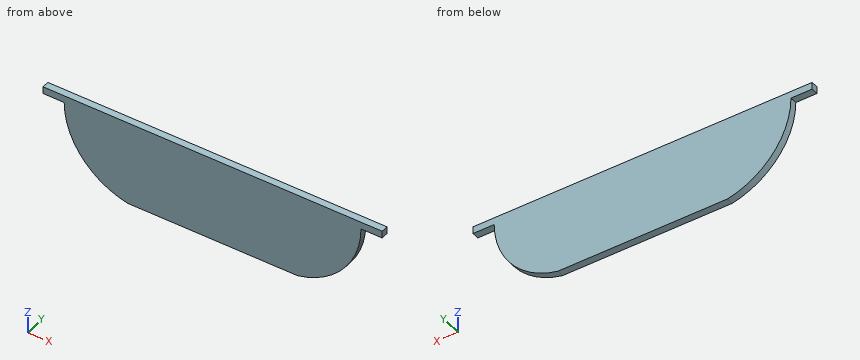
```python
from build123d import *

# Parameters (mm, degrees)
F1_DEPTH = 6.35


with BuildPart() as f1:
    # F0 (on Front) → F1 (new body)
    with BuildSketch(Plane.XZ):
        with BuildLine():
            Line((-72.007763, 0), (-97.407763, 0))
            Line((-97.407763, 0), (-97.407763, -6.35))
            Line((-97.407763, -6.35), (-78.357763, -6.35))
            ThreePointArc((-78.357763, -6.35), (-62.249709, -51.475229), (-21.207763, -76.2))
            Line((-21.207763, -76.2), (131.192237, -76.2))
            ThreePointArc((131.192237, -76.2), (172.234183, -51.475229), (188.342237, -6.35))
            Line((188.342237, -6.35), (207.392237, -6.35))
            Line((207.392237, -6.35), (207.392237, 0))
            Line((207.392237, 0), (181.992237, 0))
            Line((181.992237, 0), (54.992237, 0))
            Line((54.992237, 0), (-72.007763, 0))
        make_face()
    extrude(amount=F1_DEPTH)


solid = f1.part
```
Can you work these out from the model? Positions are in its coordinate system, mm. Give positions to 0.01 mm unless a question says otherwise; leave off trailing zeros. Order: outer loops, then holes, each group sorted by start corner. A loop starts at its lowest first (then second) coordinate and runs counter-clockwise, first axis right, second up. Notation, with made-up numbers: M 19.25,79.5 L 36.25,79.5 A5 cw 36.25,83.5 Z; hole C -5.5,-10 d2. An arc over 180 degrees is marked long. Write item = value, one per line. Start each with the question number.
Q1. Suppose I cut it at C-C (x = 173). Write out the boundary of the cut face in (y, z).
Q2. I need wall thicknesses on probe 1 along X at (y, z) = (-5.5, -7); probe 2 along X at (y, z) = (-1.5, -47); probe 3 along Z at (x, y) = (162, -1.75). Which ranges of each line are inside material? Lowest first, please. Write a range as [from, to].
Q3. Will these pins go through, and if not, where does the flat tip stop? pin 1 Ø1.9 at (x, y) = (201.5, -3) entering from -Z; pin 2 Ø2 at (y, z) = (-4.5, -26.5) entering from -X; pin 3 Ø3 at (x, y) = (-24, -3) entering from -Z.
Q4. Suppose I cut it at A-A (y = -2.75). Write out the boundary of the cut face in (x, z), plus the area to 3 significant figures.
Q5. Suppose I cut it at B-B (z = -32.5). Write out the boundary of the cut face in (x, y).
Check result:
q1.outline = M -6.35,-50.52 L 0,-50.52 L 0,0 L -6.35,0 Z
q2.probe_1 = [-78.35, 188.34]
q2.probe_2 = [-65.63, 175.61]
q2.probe_3 = [-61.67, 0]
q3.pin_1 = -6.35
q3.pin_2 = -75.74
q3.pin_3 = -75.93
q4.outline = M -97.41,-6.35 L -78.36,-6.35 A71.26 ccw -21.21,-76.2 L 131.19,-76.2 A71.26 ccw 188.34,-6.35 L 207.39,-6.35 L 207.39,0 L -97.41,0 Z
q4.area = 18,600 mm2
q5.outline = M -73.39,-6.35 L 183.37,-6.35 L 183.37,0 L -73.39,0 Z
